```python
from build123d import *

# Parameters (mm, degrees)
BOSS_EXTRUDE2_DEPTH = 1.7
FILLET2_R           = 1
SKETCH2_W           = 7
SKETCH2_H           = 3
SKETCH2_W_2         = 3
SKETCH2_H_2         = 7
SKETCH2_W_3         = 4
SKETCH2_H_3         = 4
SKETCH2_W_4         = 11
SKETCH2_H_4         = 11
BOSS_EXTRUDE3_DEPTH = 2.5
SKETCH3_W           = 11
SKETCH3_H           = 4.5
BOSS_EXTRUDE4_DEPTH = 3.7
SKETCH4_W           = 14
SKETCH4_H           = 4
BOSS_EXTRUDE5_DEPTH = 9


with BuildPart() as part:
    # Sketch1 → Boss-Extrude2 (new body)
    with BuildSketch(Plane(origin=(0, 0, 0), x_dir=(1, 0, 0), z_dir=(0, 1, 0))):
        Polygon((0, 5), (3, 5), (3, 0), (50, 0), (50, 25), (47, 25), (47, 30), (0, 30), align=None)
    extrude(amount=BOSS_EXTRUDE2_DEPTH)

    # Fillet2
    fillet2_edges = [part.edges().sort_by_distance(p)[0] for p in [
        (47, 0.85, -25),
        (3, 0.85, -5),
    ]]
    fillet(fillet2_edges, radius=FILLET2_R)

    # Sketch2 → Boss-Extrude3 (add)
    with BuildSketch(Plane(origin=(0, 1.7, 0), x_dir=(1, 0, 0), z_dir=(0, 1, 0))):
        with Locations((14.5, 28.5)):
            Rectangle(SKETCH2_W, SKETCH2_H)
        with Locations((17.5, 23.4)):
            Rectangle(SKETCH2_W_2, SKETCH2_H_2)
        with Locations((24, 7)):
            Rectangle(SKETCH2_W_3, SKETCH2_H_3)
        with Locations((36.5, 12.5)):
            Rectangle(SKETCH2_W_4, SKETCH2_H_4)
    extrude(amount=BOSS_EXTRUDE3_DEPTH)

    # Sketch3 → Boss-Extrude4 (add)
    with BuildSketch(Plane(origin=(0, 1.7, -31.7), x_dir=(-1, 0, 0), z_dir=(0, 1, 0))):
        with Locations((-38.5, 3.95)):
            Rectangle(SKETCH3_W, SKETCH3_H)
    extrude(amount=BOSS_EXTRUDE4_DEPTH)

    # Sketch4 → Boss-Extrude5 (add)
    with BuildSketch(Plane(origin=(50, 0, 0), x_dir=(0, 0, -1), z_dir=(1, 0, 0))):
        with Locations((18, 2)):
            Rectangle(SKETCH4_W, SKETCH4_H)
    extrude(amount=BOSS_EXTRUDE5_DEPTH)


solid = part.part
```
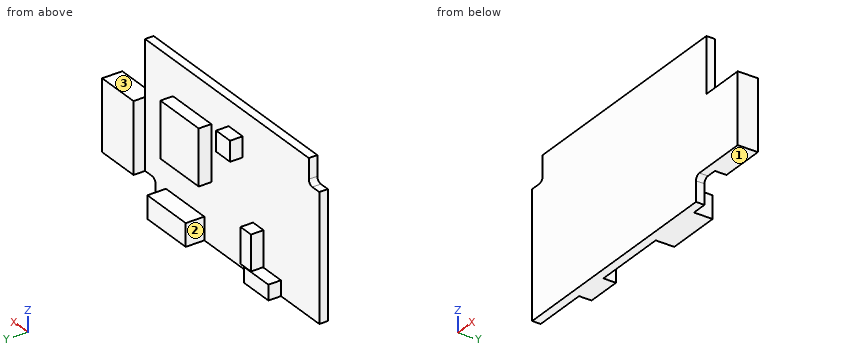
Geometry check sheet. Reference: the model listing, model coordinates, mm. Face numbers are marked on the shaded views. A direction names the side the tool comes from. Round coordinates to 2 decimals unless told otherwise and drop trailing zeros. Loops run counter-clockwise (first coordinate to the right, second up) from the corner with the lowest first, then second, coordinate; pieces in that order, holes last. Notation, with made-up numbers: (59, -23.75) - (79, -23.75) arc R11 cw to (79, -8.75) - close; hole circle Ø1 at (51.25, 53). An arc over 180 degrees is marked (long way). Write item = value, one per line. Start each with the question number.
1. Section check C-C on z = -12.5. Enter the section's corners in (x, y), then the cut area to 4 significant figures.
2. Depth check by flat-ended pin: pin 1 (3 mm diameter, centred on y = 4, z = -28.5, fed in from -X); pin 2 (1.4 mm diameter, centred on y = 1, z = -3.5, fed in from +X); pin 3 (1.2 mm diameter, centred on x = 24.5, y = 3, fed in from +Z). Enter the tip coordinate at first touch or a pass-through.
3. Set-up check for the marked faces 1, 2 and 3: record each of +Z, -Z, +X, -X, +Y, -Y from which the full face is reachable in a straight line by a thin tool's end or side.
4. Section check A-A on z = -22.25. Enter the section's corners in (x, y).
5. Section check B-B on x = 52.5. Enter the section's corners in (y, z).
6. Thickness scan on line 1 (Z direction, x = 40, y = 3.6); line 2 (X direction, y = 2.65, z = -13); line 3 (Z direction, x = 51, y = 0.4). Record the ranges inside material, lowest first.
Working result:
q1.outline = (0, 0) - (59, 0) - (59, 4) - (50, 4) - (50, 1.7) - (42, 1.7) - (42, 4.2) - (31, 4.2) - (31, 1.7) - (0, 1.7) - close
q1.area = 148.5 mm^2
q2.pin_1 = 11
q2.pin_2 = 50
q2.pin_3 = -5
q3.face_1 = -Z, +X, +Y, -Y
q3.face_2 = -Z, +Y
q3.face_3 = +Z, +X, +Y, -Y
q4.outline = (0, 0) - (59, 0) - (59, 4) - (50, 4) - (50, 1.7) - (19, 1.7) - (19, 4.2) - (16, 4.2) - (16, 1.7) - (0, 1.7) - close
q5.outline = (0, -25) - (4, -25) - (4, -11) - (0, -11) - close
q6.line_1 = -30 to -25.5, -18 to -7
q6.line_2 = 31 to 42, 50 to 59
q6.line_3 = -25 to -11
